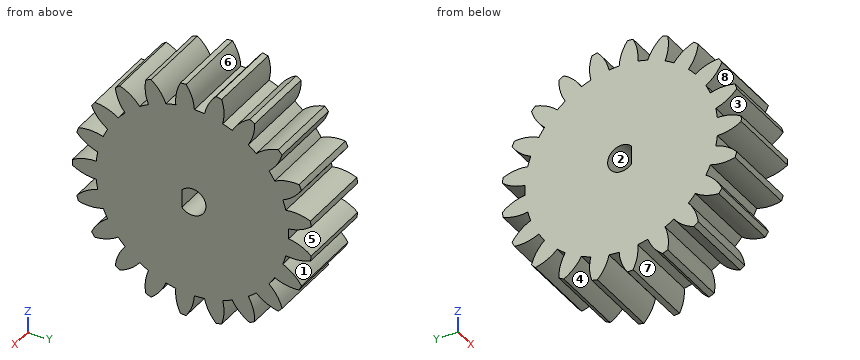
```python
from build123d import *

# Parameters (mm, degrees)
BASPROSKE_W         = 15
BASPROSKE_H         = 23
TOOTHCUT_DEPTH      = 36.818989377
TEETHCUTS_COUNT     = 21
TEETHCUTS_ANGLE     = 342.857142857
BORSKE_R            = 2.5
BORE_DEPTH          = 50.0000508
SKETCH_1_R          = 2.625
CUT_EXTRUDE_1_DEPTH = 15
SKETCH_3_W          = 3.458323293
SKETCH_3_H          = 0.848920995
EXTRUDE_1_DEPTH     = 15


with BuildPart() as part:
    # BasProSke → Base-Revolve (revolve)
    with BuildSketch(Plane(origin=(0, 0, 0), x_dir=(1, 0, 0), z_dir=(0, 1, 0)), mode=Mode.PRIVATE) as base_revolve_sk:
        with Locations((7.5, 11.5)):
            Rectangle(BASPROSKE_W, BASPROSKE_H)
    revolve(base_revolve_sk.sketch.rotate(Axis((-10, 0, 0), (1, 0, 0)), 180), axis=Axis((-10, 0, 0), (1, 0, 0)))

    # TooCutSke → ToothCut (cut, through all)
    with BuildSketch(Plane(origin=(0, 0, 0), x_dir=(0, 0, -1), z_dir=(1, 0, 0))):
        with BuildLine():
            ThreePointArc((0.976779145, 18.473194188), (0, 18.499), (-0.976779145, 18.473194188))
            ThreePointArc((-0.976779145, 18.473194188), (-1.625451341, 20.797249275), (-2.90802115, 22.841025768))
            ThreePointArc((-2.90802115, 22.841025768), (0, 23.0254), (2.90802115, 22.841025768))
            ThreePointArc((2.90802115, 22.841025768), (1.625451341, 20.797249275), (0.976779145, 18.473194188))
        make_face()
    toothcut = extrude(amount=TOOTHCUT_DEPTH, mode=Mode.SUBTRACT)

    # TeethCuts: ToothCut ×21 about axis
    teethcuts_axis = Axis((-10, 0, 0), (1, 0, 0))
    for i in range(1, TEETHCUTS_COUNT):
        add(toothcut.rotate(teethcuts_axis, i * TEETHCUTS_ANGLE / (TEETHCUTS_COUNT - 1)), mode=Mode.SUBTRACT)

    # BorSke → Bore (cut, symmetric)
    with BuildSketch(Plane(origin=(0, 0, 0), x_dir=(0, 0, -1), z_dir=(1, 0, 0))):
        with Locations(Location((0, 0, 0), (0, 0, 180))):
            Circle(BORSKE_R)
    extrude(amount=BORE_DEPTH, both=True, mode=Mode.SUBTRACT)

    # 草圖1 → 除料-伸長1 (cut)
    with BuildSketch(Plane.ZY):
        Circle(SKETCH_1_R)
    extrude(amount=-CUT_EXTRUDE_1_DEPTH, mode=Mode.SUBTRACT)

    # 草圖3 → 填料-伸長1 (add)
    with BuildSketch(Plane.ZY):
        with Locations((0.024656151, -2.399460498)):
            Rectangle(SKETCH_3_W, SKETCH_3_H)
    extrude(amount=-EXTRUDE_1_DEPTH)


solid = part.part
```
For this review, take the finished solid that the model builds, in its own axes (mm). Face numbers are marked on the shaded views. A direction names the side the tool comes from. Round coordinates to 2 decimals unless told otherwise and drop trailing zeros. Write each loop counter-clockwise with the first axis right and the second up, starting at its lowest first coordinate (ties: lowest second). Pieces come first, ordered by that corner, then holes. Notation, with made-up numbers: (-21.5, 80) -> (22.5, 80) arc R13 ccw to (22.5, 99) -> close; hole circle Ø10 at (-15, -20). An arc over 180 degrees is marked (long way). One line per question, with ' | ' between items. Start each with the question number.
(1) For line 1 along Z through (x, y) = (9.75, -19); line 2 along Y through (x, z) = (12, 20); line 3 along Z through (x, y) = (2, 15), list the stretches that pass through material, from the lowest coordinate up. Write a range as from..to.
(2) Insertion check: P1, Ø6, axis at x = 4, y = 15.5, coming from the -Z side; P2, Ø6, axis at x = 8.5, z = 13, coming from the +Y side; P3, Ø4, axis at x = 5, y = 7, coming from the +Z side. Each pin has a flat end and moves straight along its axis. Give the tip position at first contact, or say it passes through.
(3) Add section A-A, the plane z = 0. Write out the cut boundary in (x, y) (3 decimals), plus the area to 3 significant figures.
(4) Tool access review of the marked faces 4, 5, 6, 7 and 8: name each direction out of +Z, -Z, +X, -X, +Y, -Y from which nothing blocks a thin tool from reaching the whole face with its end or side.
(5) Mouldability with a two-part tool opening along Y and no side actions: class the marked faces 1, 2 and 3 as released by +Y, released by -Y, zero draft, split by the parting line, or undercut.
(6) Add section B-B, the plane y = -6.5. Write out the cut boundary in (x, z).
Answer list:
1) line 1: -12.96..-11.89, -7.53..-4.02, -1.78..1.78, 4.02..7.53, 11.89..12.96 | line 2: -9.03..-6.28, -3.14..0.19, 2.88..6.08, 10.7..11.36 | line 3: -15.6..-11.48, -10.83..10.83, 11.48..15.6
2) P1: z = -16.04 | P2: y = 20.71 | P3: z = 22.45
3) outline: (0, -23) -> (15, -23) -> (15, -1.975) -> (0, -1.975) -> close; (0, 2.625) -> (15, 2.625) -> (15, 18.499) -> (0, 18.499) -> close | area: 553 mm²
4) face 4: -Z, +X, -X | face 5: +X, -X, +Y | face 6: +Z, +X, -X | face 7: +X, -X | face 8: +X, -X, -Y
5) face 1: released by +Y | face 2: undercut | face 3: released by -Y
6) outline: (0, -20.28) -> (15, -20.28) -> (15, 20.28) -> (0, 20.28) -> close
